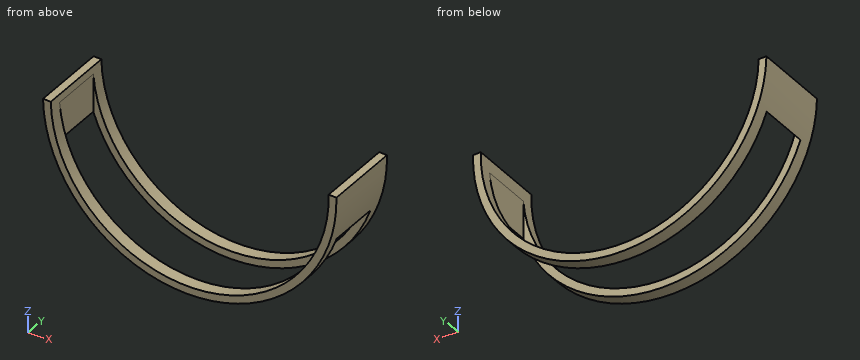
from build123d import *

# Parameters (mm, degrees)
BOSS_EXTRUDE1_DEPTH     = 15
CUT_EXTRUDE1_DEPTH      = 82.515026332
CUT_EXTRUDE1_DEPTH_BACK = 200
SKETCH3_W               = 107
SKETCH3_H               = 20


with BuildPart() as part:
    # Sketch1 → Boss-Extrude1 (new, symmetric)
    with BuildSketch(Plane(origin=(0, 0, 0), x_dir=(1, 0, 0), z_dir=(0, 1, 0))):
        with BuildLine():
            Line((-56.6451424, 1.085173475), (-53.646875163, 1.186754079))
            ThreePointArc((-53.646875163, 1.186754079), (1.186754079, 53.646875163), (53.646875163, -1.186754079))
            Line((53.646875163, -1.186754079), (56.645146911, -1.084937955))
            ThreePointArc((56.645146911, -1.084937955), (1.085055715, 56.645144656), (-56.6451424, 1.085173475))
        make_face()
    extrude(amount=BOSS_EXTRUDE1_DEPTH, both=True)

    # Sketch3 → Cut-Extrude1 (cut, two sides: drawn at the far end of the back side and taken through both)
    with BuildSketch(Plane.XY.offset(-CUT_EXTRUDE1_DEPTH_BACK)):
        Rectangle(SKETCH3_W, SKETCH3_H)
    extrude(amount=CUT_EXTRUDE1_DEPTH + CUT_EXTRUDE1_DEPTH_BACK, mode=Mode.SUBTRACT)


solid = part.part
Verification items for the finished model (mm, model axes). Give positions to 0.01 mm unless a question says otherwise; leave off trailing zeros. Write each loop counter-clockwise with the first axis right and the second up, starting at its lowest first coordinate (ties: lowest second). Pieces come first, ordered by that corner, then holes. Notation, with made-up numbers: M 3.25,-14 L 39.25,-14 A34 ccw 39.25,25 Z; hole C -23.5,-4.75 d3. An arc over 180 degrees is marked long. Write item = value, one per line.
(1) Go/stop test with flat-tipped pins: pin 1 Ø16 at (y, z) = (0.5, -15) entering from +X; pin 2 Ø8 at (x, y) = (8.5, -8) entering from +Z; pin 3 Ø2 at (x, y) = (-16.5, -12) entering from -Z. Record where each tip stops, or that it passes through.
Found:
pin_1 = 56.22
pin_2 = -52.31
pin_3 = -54.49
(2) Sectioned sample at B-B (x = 0). Record the cut outline in (y, z).
Found:
outline = M -15,-56.66 L -10,-56.66 L -10,-53.66 L -15,-53.66 Z; M 10,-56.66 L 15,-56.66 L 15,-53.66 L 10,-53.66 Z
(3) Sectioned sample at C-C (z = -47.5). Record the cut outline in (x, y).
Found:
outline = M -30.88,-15 L -24.96,-15 L -24.96,-10 L -30.88,-10 Z; M -30.88,10 L -24.96,10 L -24.96,15 L -30.88,15 Z; M 24.96,-15 L 30.88,-15 L 30.88,-10 L 24.96,-10 Z; M 24.96,10 L 30.88,10 L 30.88,15 L 24.96,15 Z
(4) Sectioned sample at D-D (z = -11.5). Record the cut outline in (x, y).
Found:
outline = M -55.48,-15 L -52.41,-15 L -52.41,-10 L -53.5,-10 L -53.5,10 L -52.41,10 L -52.41,15 L -55.48,15 Z; M 52.41,-15 L 55.48,-15 L 55.48,15 L 52.41,15 L 52.41,10 L 53.5,10 L 53.5,-10 L 52.41,-10 Z
(5) Material ranges on line 1 (X direction, y = -12.25, z = -28); line 2 (X direction, y = 7.5, z = -9.5); line 3 (Z direction, x = 4, y = -12.5), recorded low to high.
Found:
line_1 = -49.25 to -45.78, 45.78 to 49.25
line_2 = -55.85 to -53.5, 53.5 to 55.85
line_3 = -56.51 to -53.51
(6) Sectioned sample at A-A (y = -3.25). Record the cut outline in (x, z).
Found:
outline = M -56.65,-1.09 A56.66 ccw -53.5,-18.64 L -53.5,-4.14 A53.66 cw -53.65,-1.19 Z; M 53.5,-18.64 A56.66 ccw 56.65,1.08 L 53.65,1.19 A53.66 cw 53.5,-4.14 Z
